Source: CAD feature listing. Evaluate the final solid. Frame: model axes, mm. A direction names the side the tool comes from. Give positions to 0.01 mm unless a question says otherwise; leave off trailing zeros. Loops run counter-clockwise (first coordinate to the right, second up) from the corner with the lowest first, then second, coordinate; pieces in that order, holes last. Notation, with made-up numbers: M 66.25,5.25 L 102.25,5.25 A23 cw 102.25,36.25 Z; hole C 3,70.25 d5. An arc over 180 degrees is marked long. Put each result on its own line as item: value. Start each with the question number.
```python
from build123d import *

# Parameters (mm, degrees)
BOSS_EXTRUDE1_DEPTH           = 76.2
TAP_DRILL_FOR_8_36_TAP1_D     = 3.4544
TAP_DRILL_FOR_8_36_TAP2_D     = 3.4544
TAP_DRILL_FOR_8_36_TAP2_DEPTH = 3.175


with BuildPart() as part:
    # Sketch1 → Boss-Extrude1 (new body)
    with BuildSketch(Plane.XY):
        Polygon((0, 0), (0, 28.575), (-28.575, 28.575), (-28.575, 25.4), (-3.175, 25.4), (-3.175, 0), align=None)
    extrude(amount=BOSS_EXTRUDE1_DEPTH)

    # Tap Drill for #8-36 Tap1 (through all)
    with Locations(Plane.ZY.offset(3.175)):
        with Locations((38.1, 6.6), (38.1, 19.3)):
            Hole(TAP_DRILL_FOR_8_36_TAP1_D / 2)

    # Tap Drill for #8-36 Tap2
    with Locations(Plane(origin=(0, 25.4, 0), x_dir=(-1, 0, 0), z_dir=(0, -1, 0))):
        with Locations((9.525, -63.5), (-28.575, -63.5), (9.525, -13.711593905), (-28.575, -13.711593905)):
            Hole(TAP_DRILL_FOR_8_36_TAP2_D / 2, depth=TAP_DRILL_FOR_8_36_TAP2_DEPTH)


solid = part.part
```
1. Contact query for flat-ended pins moving along their axis: pin 1 (2 mm diameter, centred on x = -14.5, z = 32, fed in from -Y); pin 2 (10 mm diameter, centred on y = 16, z = 47.5, fed in from -X) (3 decimals). Output: stop coordinate, or through.
2. Section A-A, the plane z = 63.5. Output: boundary loops of the cut face in (x, y) (3 decimals).
3. Ray query, line 1 (Y direction, x = -0.9, z = 38.1) (3 decimals); line 2 (X direction, y = 27.75, z = 63.5) (3 decimals); line 3 (Y direction, x = -25.25, z = 4) (3 decimals). Return the intervals inside material, ascending.
4. Set-up query: faces 1 (the face through (-9, 26, 0)), 2 (the face through (-3.175, 13, 38)). Return all of +Z, -Z, +X, -X, +Y, -Y with unobstructed straight access to the full face (end or side cutting, diameter ignored); none if empty.
5. Section B-B, the plane z = 38.1. Output: boundary loops of the cut face in (x, y) (3 decimals), plus the area to 3 significant figures.
6. Section C-C, the plane y = 19.3. Output: boundary loops of the cut face in (x, z) (3 decimals).
7. Pull-direction query (Y, two-part tool) for faces 3 (the face through (-1.565, 6.676, 39.826)), 4 (the face through (-7.88, 27.01, 13.19)), 5 (the face through (-16, 25.4, 38)); classes: released by +Y, released by -Y, zero draft, split by the parting line, or undercut.
8. Section D-D, the plane x = -15. Output: boundary loops of the cut face in (y, z) (3 decimals), plus the area to 3 significant figures.
Results found:
1. pin 1: y = 25.4
1. pin 2: x = -3.175
2. outline: M -28.575,25.4 L -11.252,25.4 L -11.252,28.575 L -28.575,28.575 Z; M -7.798,25.4 L -3.175,25.4 L -3.175,0 L 0,0 L 0,28.575 L -7.798,28.575 Z
3. line 1: 0 to 4.873, 8.327 to 17.573, 21.027 to 28.575
3. line 2: -28.575 to -11.252, -7.798 to 0
3. line 3: 25.4 to 28.575
4. face 1: -Z, +X, -X, +Y, -Y
4. face 2: +Z, -Z, -X, -Y
5. outline: M -28.575,25.4 L -3.175,25.4 L -3.175,21.027 L 0,21.027 L 0,28.575 L -28.575,28.575 Z; M -3.175,0 L 0,0 L 0,4.873 L -3.175,4.873 Z; M -3.175,8.327 L 0,8.327 L 0,17.573 L -3.175,17.573 Z
5. area: 149 mm²
6. outline: M -3.175,0 L 0,0 L 0,36.373 L -3.175,36.373 Z; M -3.175,39.827 L 0,39.827 L 0,76.2 L -3.175,76.2 Z
7. face 3: undercut
7. face 4: zero draft
7. face 5: released by -Y
8. outline: M 25.4,0 L 28.575,0 L 28.575,76.2 L 25.4,76.2 Z
8. area: 242 mm²
